Could you check a few things on this model? Use its own coordinates, in mm. A direction names the side the tool comes from. Give positions to 0.01 mm unless a question says otherwise; leave off trailing zeros. Loops run counter-clockwise (first coordinate to the right, second up) from the corner with the lowest first, then second, coordinate; pieces in that order, holes last.
1. For faces 1 (the cylindrical face through (-29.97, -1.32, -115.11)), 2 (the flat face through (0, 0, -165.5)), which set-ups out of +Z, -Z, +X, -X, +Y, -Y let a thin tool reach every point of the face, with its end or its side?
2. Imagine slicing it at C-C (x = 2). List the corners of the cut face in (y, z) for me.
3. I need wall thicknesses on line 1 along Z through (x, y) = (-30.5, -10.5); line 2 along Z through (x, y) = (13, -17.5); line 3 along Y through (x, z) = (3, 77.5). Which ranges of each line are inside material? Lowest first, please.
4. Imagine slicing it at D-D (y = 27). List the corners of the cut face in (x, z) for me.
5. Imagine slicing it at B-B (x = -26.5). List the corners of the cut face in (y, z) for me, plus the area to 3 significant figures.
6. For P1, Ø8, axis at x = -29, y = 20, coming from the -Z side; P2, Ø1, axis at y = -15, z = -117.5, coming from the +X side; P3, Ø3, axis at x = 16, z = -49, coming from the +Y side, each with a flat end and sliding along its axis, tell me the tip position at first contact or that it passes through.
7. Imagine slicing it at A-A (y = 0). List the corners of the cut face in (x, z) for me, plus the area to 3 significant figures.
```python
from build123d import *

# Parameters (mm, degrees)
F0_R     = 40
F1_DEPTH = 105
F2_R     = 30
F3_DEPTH = 20.5
F4_R     = 15
F5_DEPTH = 40


with BuildPart() as f1:
    # F0 (on Top) → F1 (new body, symmetric)
    with BuildSketch(Plane.XY):
        with Locations((1.18393, 0)):
            Circle(F0_R)
    extrude(amount=F1_DEPTH, both=True)

    # F2 (on face) → F3 (join)
    with BuildSketch(Plane(origin=(0, 0, -105), x_dir=(1, 0, 0), z_dir=(0, 0, -1))):
        Circle(F2_R)
    extrude(amount=F3_DEPTH)

    # F4 (on face) → F5 (join)
    with BuildSketch(Plane(origin=(0, 0, -125.5), x_dir=(1, 0, 0), z_dir=(0, 0, -1))):
        Circle(F4_R)
    extrude(amount=F5_DEPTH)


solid = f1.part
```
Derived:
1. face 1: -Z
1. face 2: -Z, +X, -X, +Y, -Y
2. outline: (-39.99, -105) - (-29.93, -105) - (-29.93, -125.5) - (-14.87, -125.5) - (-14.87, -165.5) - (14.87, -165.5) - (14.87, -125.5) - (29.93, -125.5) - (29.93, -105) - (39.99, -105) - (39.99, 105) - (-39.99, 105) - close
3. line 1: z = -105 to 105
3. line 2: z = -125.5 to 105
3. line 3: y = -39.96 to 39.96
4. outline: (-28.33, -105) - (-13.08, -105) - (-13.08, -125.5) - (13.08, -125.5) - (13.08, -105) - (30.7, -105) - (30.7, 105) - (-28.33, 105) - close
5. outline: (-28.87, -105) - (-14.06, -105) - (-14.06, -125.5) - (14.06, -125.5) - (14.06, -105) - (28.87, -105) - (28.87, 105) - (-28.87, 105) - close
5. area: 12,700 mm2
6. P1: stops at z = -105
6. P2: stops at x = 26.26
6. P3: stops at y = 37.72
7. outline: (-38.82, -105) - (-30, -105) - (-30, -125.5) - (-15, -125.5) - (-15, -165.5) - (15, -165.5) - (15, -125.5) - (30, -125.5) - (30, -105) - (41.18, -105) - (41.18, 105) - (-38.82, 105) - close
7. area: 19,200 mm2
